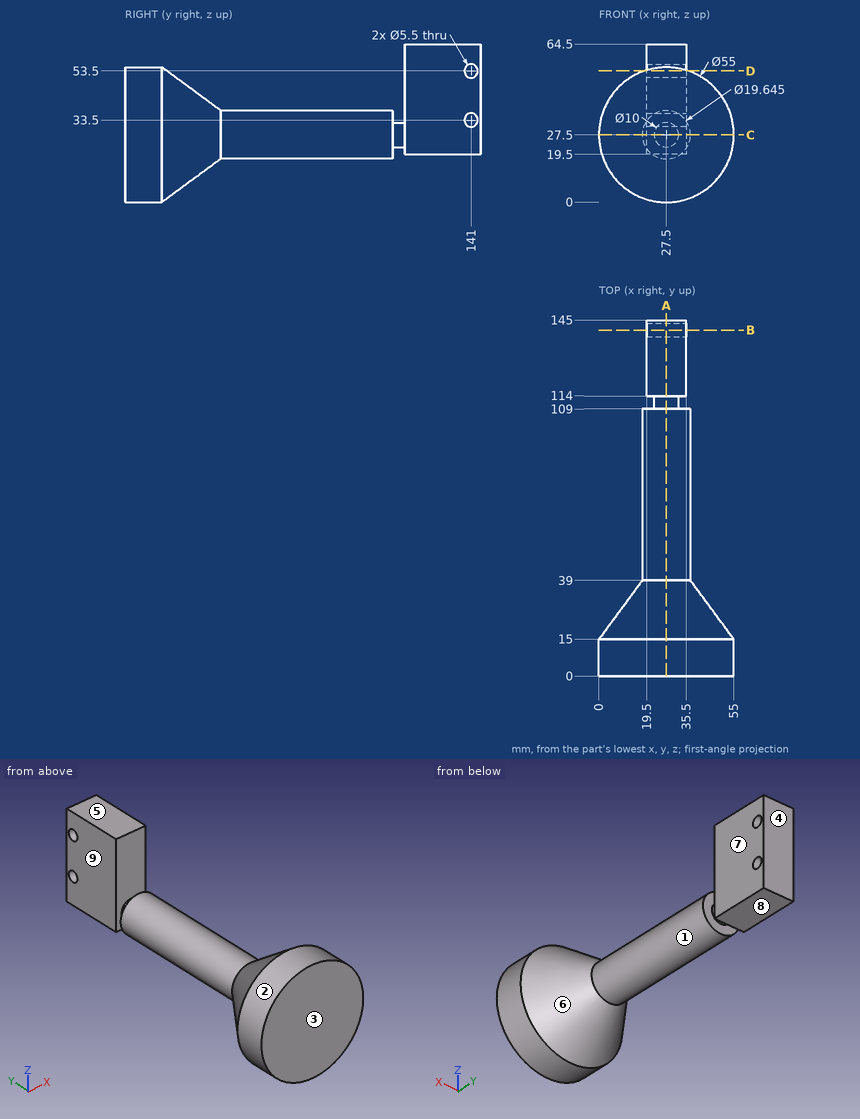
Source: three-view drawing plus pictorial views. Frame: mm from the lowest corner of the part. A direction names the side the tool comes from. Round coordinates to 2 decimals unless told otherwise and drop trailing zeros. Order: outer loops, then holes, each group sorted by start corner. A loop starts at its lowest first (then second) coordinate and runs counter-clockwise, first axis right, second up. Notation, with made-up numbers: (83.5, -13) - (106.5, -13) arc R20 cw to (106.5, 6) - close; hole circle Ø7 at (51, 12.25). An arc over 180 degrees is marked (long way). Use a Markdown table: item, result.
1. Mould query, pull axis Y, two halves, no side actions, for the marked faces 1, 2, 3 and 4. Classes: +Y half, -Y half, draft (parallel to the pull), parting line (faces both ways), or undercut.
Evaluation:
| item | result |
|---|---|
| face 1 | undercut |
| face 2 | draft |
| face 3 | -Y half |
| face 4 | +Y half |
2. First-contact query: pin 1 (5 mm diameter, centred on y = 126.5, z = 18, fed in from -X); pin 2 (8 mm diameter, centred on x = 24, z = 51.5, fed in from -Y); pin 3 (9 mm diameter, centred on y = 141, z = 33.5, fed in from +X); pin 4 (17.5 mm diameter, centred on x = 27, y = 125.5, fed in from -Z). Flat tips, straight axial feed; report the tip coordinate or a pass-through.
Evaluation:
| item | result |
|---|---|
| pin 1 | x = 19.5 |
| pin 2 | y = 0 |
| pin 3 | x = 35.5 |
| pin 4 | z = 19.5 |
3. Access query for the marked faces 5, 6, 7, 8 and 9. Directions: +Z, -Z, +X, -X, +Y, -Y. A direction counts if a zero-diameter tool reaches every point of the face in a straight line with its end or side. Return the directions, or none.
Evaluation:
| item | result |
|---|---|
| face 5 | +Z, +X, -X, +Y, -Y |
| face 6 | none |
| face 7 | +Z, -Z, +X, +Y |
| face 8 | -Z, +X, -X, +Y |
| face 9 | +Z, -Z, -X, +Y |
4. Section D-D on z = 53.5. State how many separate pieces and enclosed holes the cut face has, then the cut area to 3 significant figures.
Evaluation:
| item | result |
|---|---|
| separate pieces | 3 |
| enclosed holes | 0 |
| area | 701 mm^2 |
5. Section A-A on x = 27.5. Return the cut outline in (y, z).
Evaluation:
| item | result |
|---|---|
| outline | (0, 0) - (15, 0) - (39, 17.68) - (109, 17.68) - (109, 22.5) - (114, 22.5) - (114, 19.5) - (145, 19.5) - (145, 64.5) - (114, 64.5) - (114, 32.5) - (109, 32.5) - (109, 37.32) - (39, 37.32) - (15, 55) - (0, 55) - close; hole circle Ø5.5 at (141, 33.5); hole circle Ø5.5 at (141, 53.5) |
6. Section B-B on y = 141. Return the cut outline in (x, z), then the cut area to 3 significant figures.
Evaluation:
| item | result |
|---|---|
| outline | (19.5, 19.5) - (35.5, 19.5) - (35.5, 30.75) - (19.5, 30.75) - close; (19.5, 36.25) - (35.5, 36.25) - (35.5, 50.75) - (19.5, 50.75) - close; (19.5, 56.25) - (35.5, 56.25) - (35.5, 64.5) - (19.5, 64.5) - close |
| area | 544 mm^2 |
7. Material intervals for probe 1 along Z at (x, y) = (27.5, 141); probe 2 along Y at (x, z) = (31, 53.5); probe 3 along Y at (x, z) = (28, 53.5), sorted ascending.
Evaluation:
| item | result |
|---|---|
| probe 1 | 19.5 to 30.75, 36.25 to 50.75, 56.25 to 64.5 |
| probe 2 | 0 to 16.72, 114 to 138.25, 143.75 to 145 |
| probe 3 | 0 to 17.03, 114 to 138.25, 143.75 to 145 |
8. Section C-C on z = 27.5. Return the cut outline in (x, y), then the cut area to 3 significant figures.
Evaluation:
| item | result |
|---|---|
| outline | (0, 0) - (55, 0) - (55, 15) - (37.32, 39) - (37.32, 109) - (32.5, 109) - (32.5, 114) - (35.5, 114) - (35.5, 145) - (19.5, 145) - (19.5, 114) - (22.5, 114) - (22.5, 109) - (17.68, 109) - (17.68, 39) - (0, 15) - close |
| area | 3,640 mm^2 |
